Part model, mm, in its own coordinate system. A direction names the side the tool comes from. Round coordinates to 2 decimals unless told otherwise and drop trailing zeros. Write each loop counter-clockwise with the first axis right and the second up, starting at its lowest first coordinate (ties: lowest second). Pieces come first, ordered by that corner, then holes.
1) Saw through at C-C on x = 11. Write the cut outline in (y, z).
2) Drill centre lines: L1, parallel to Z at x = 11, y = 0.5; L2, parallel to Y at x = -2, z = 0.25; L3, parallel to X at y = -1, z = -2. Where is each one in solid material? Low to high.
3) Saw through at B-B on y = -3. Write the cut outline in (x, z).
4) Which spindle directions (+Z, -Z, +X, -X, +Y, -Y) get a long thin tool onto all of the face, cutting with end or side? Do faces 4 (the flat face through (11, 1, -7)), 5 (the flat face through (2, 5, 0)), 6 (the flat face through (9.216, -3.521, 2.989)). Say none if no direction does.
5) Flat gauge pins, fed straight in: pin 1 (2 mm diameter, centred on x = 5, z = -4.5, fed in from +Y); pin 2 (1.6 mm diameter, centred on y = 6, z = 1.5, fed in from -X); pin 3 (2 mm diameter, centred on x = 12, z = -4.5, fed in from -Y). Where does each tip first touch, or does it go through?
6) Saw through at A-A on z = 0. Write the cut outline in (x, y), and give its area (3 significant figures).
7) Saw through at D-D on x = -2.25. Write the cut outline in (y, z).
8) Pull direction Z, two halves, no side cores. Call faces 1 (the flat face through (11, 1, 7)), 2 (the cylindrical face through (-5, -4, 0)), 3 (the cylindrical face through (-1.552, 3.732, -0.345)): +Z half, -Z half, draft (parallel to the pull), parting line (faces both ways), or undercut.
```python
from build123d import *

# Parameters (mm, degrees)
BOSS_EXTRUDE1_DEPTH      = 7
BOSS_EXTRUDE1_DEPTH_BACK = 5
SKETCH1_W                = 8
SKETCH1_H                = 14
BOSS_EXTRUDE2_START      = 2.5
SKETCH1_3_R              = 1.59
BOSS_EXTRUDE2_DEPTH      = 2.5
BOSS_EXTRUDE3_START      = -5
SKETCH1_4_R              = 1.59
BOSS_EXTRUDE3_DEPTH      = 2.5
M2_CLEARANCE_HOLE1_D     = 2.6
CUT_EXTRUDE1_DEPTH       = 3
FILLET2_R                = 1


with BuildPart() as part:
    # Sketch1 → Boss-Extrude1 (new, two sides: drawn at the far end of the back side and taken through both)
    with BuildSketch(Plane(origin=(0, 0, 0), x_dir=(1, 0, 0), z_dir=(0, 1, 0)).offset(-BOSS_EXTRUDE1_DEPTH_BACK)):
        with Locations((11, 0)):
            Rectangle(SKETCH1_W, SKETCH1_H)
    extrude(amount=BOSS_EXTRUDE1_DEPTH + BOSS_EXTRUDE1_DEPTH_BACK)

    # Sketch1<3> → Boss-Extrude2 (add)
    with BuildSketch(Plane(origin=(0, 0, 0), x_dir=(1, 0, 0), z_dir=(0, 1, 0)).offset(BOSS_EXTRUDE2_START)):
        with BuildLine():
            Line((7, 7), (-1.265715623, 4.837144195))
            ThreePointArc((-1.265715623, 4.837144195), (-5, 0), (-1.265715623, -4.837144195))
            Line((-1.265715623, -4.837144195), (7, -7))
            Line((7, -7), (7, 7))
        make_face()
        with Locations(Location((0, 0, 0), (0, 0, 270))):
            Circle(SKETCH1_3_R, mode=Mode.SUBTRACT)
    extrude(amount=BOSS_EXTRUDE2_DEPTH)

    # Sketch1<4> → Boss-Extrude3 (add)
    with BuildSketch(Plane(origin=(0, 0, 0), x_dir=(1, 0, 0), z_dir=(0, 1, 0)).offset(BOSS_EXTRUDE3_START)):
        with BuildLine():
            Line((7, 7), (-1.265715623, 4.837144195))
            ThreePointArc((-1.265715623, 4.837144195), (-5, 0), (-1.265715623, -4.837144195))
            Line((-1.265715623, -4.837144195), (7, -7))
            Line((7, -7), (7, 7))
        make_face()
        with Locations(Location((0, 0, 0), (0, 0, 270))):
            Circle(SKETCH1_4_R, mode=Mode.SUBTRACT)
    extrude(amount=BOSS_EXTRUDE3_DEPTH)

    # M2 Clearance Hole1 (through all)
    with Locations(Plane(origin=(0, 7, 0), x_dir=(1, 0, 0), z_dir=(0, 1, 0))):
        with Locations((11, 4), (11, -4)):
            Hole(M2_CLEARANCE_HOLE1_D / 2)

    # Sketch4 → Cut-Extrude1 (cut)
    with BuildSketch(Plane.XZ.offset(5)):
        Polygon((9.816431948, 1.95), (12.183568052, 1.95), (13.367136104, 4), (12.183568052, 6.05), (9.816431948, 6.05), (8.632863896, 4), align=None)
        Polygon((8.632863896, -4), (9.816431948, -6.05), (12.183568052, -6.05), (13.367136104, -4), (12.183568052, -1.95), (9.816431948, -1.95), align=None)
    extrude(amount=-CUT_EXTRUDE1_DEPTH, mode=Mode.SUBTRACT)

    # Fillet2
    fillet2_edges = [part.edges().sort_by_distance(p)[0] for p in [
        (15, 7, 0),
    ]]
    fillet(fillet2_edges, radius=FILLET2_R)


solid = part.part
```
Completed:
1. outline: (-5, -7) - (7, -7) - (7, -5.3) - (-2, -5.3) - (-2, -6.05) - (-5, -6.05) - close; (-5, -1.95) - (-2, -1.95) - (-2, -2.7) - (7, -2.7) - (7, 2.7) - (-2, 2.7) - (-2, 1.95) - (-5, 1.95) - close; (-5, 6.05) - (-2, 6.05) - (-2, 5.3) - (7, 5.3) - (7, 7) - (-5, 7) - close
2. L1: z = -7 to -5.3, -2.7 to 2.7, 5.3 to 7
2. L2: y = -5 to -2.5, 2.5 to 5
2. L3: x = 7 to 15
3. outline: (-1.27, -4.84) - (7, -7) - (15, -7) - (15, 7) - (7, 7) - (-1.27, 4.84) arc R5 ccw to start; hole circle Ø3.18 at (0, 0); hole (8.63, -4) - (9.82, -6.05) - (12.18, -6.05) - (13.37, -4) - (12.18, -1.95) - (9.82, -1.95) - close; hole (8.63, 4) - (9.82, 1.95) - (12.18, 1.95) - (13.37, 4) - (12.18, 6.05) - (9.82, 6.05) - close
4. face 4: -Z, +X, -X, +Y, -Y
4. face 5: +Z, -Z, -X, +Y
4. face 6: -Y
5. pin 1: stops at y = 5
5. pin 2: stops at x = 7
5. pin 3: stops at y = -5
6. outline: (-5, -5) - (-1.59, -5) - (-1.59, -2.5) - (-5, -2.5) - close; (-5, 2.5) - (-1.59, 2.5) - (-1.59, 5) - (-5, 5) - close; (1.59, -5) - (15, -5) - (15, 6) arc R1 ccw to (14, 7) - (7, 7) - (7, 5) - (1.59, 5) - (1.59, 2.5) - (7, 2.5) - (7, -2.5) - (1.59, -2.5) - close
6. area: 140 mm2
7. outline: (-5, -4.47) - (-2.5, -4.47) - (-2.5, 4.47) - (-5, 4.47) - close; (2.5, -4.47) - (5, -4.47) - (5, 4.47) - (2.5, 4.47) - close
8. face 1: +Z half
8. face 2: parting line
8. face 3: undercut
